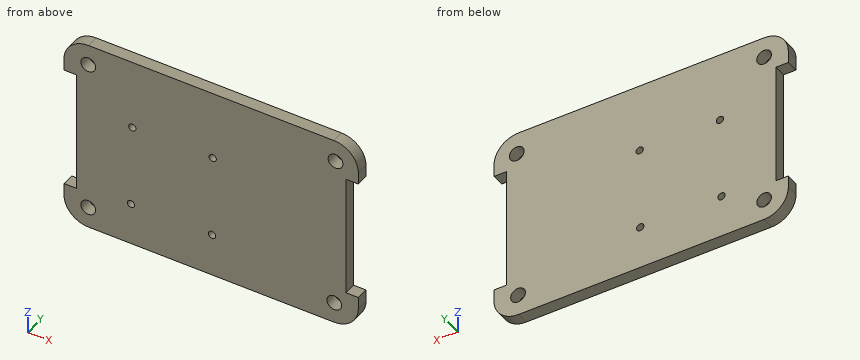
from build123d import *

# Parameters (mm, degrees)
BOSS_EXTRUDE1_DEPTH = 5
SKETCH2_R           = 3
SKETCH2_R_2         = 3.002001364
SKETCH2_R_3         = 2.999925667
SKETCH2_R_4         = 2.998527559
CUT_EXTRUDE2_DEPTH  = 5
SKETCH14_R          = 1.488706827
SKETCH14_R_2        = 1.489546346
SKETCH14_R_3        = 1.489389331
SKETCH14_R_4        = 1.489192683
CUT_EXTRUDE3_DEPTH  = 5


with BuildPart() as part:
    # Sketch1 → Boss-Extrude1 (new body)
    with BuildSketch(Plane(origin=(0, 0, 0), x_dir=(1, 0, 0), z_dir=(0, 1, 0))):
        with BuildLine():
            Line((10, 0), (110, 0))
            ThreePointArc((110, 0), (117.071067812, -2.928932188), (120, -10))
            Line((120, -10), (120, -15))
            Line((120, -15), (115, -15))
            Line((115, -15), (115, -65))
            Line((115, -65), (120, -65))
            Line((120, -65), (120, -70))
            ThreePointArc((120, -70), (117.071067812, -77.071067812), (110, -80))
            Line((110, -80), (10, -80))
            ThreePointArc((10, -80), (2.928932188, -77.071067812), (0, -70))
            Line((0, -70), (0, -65))
            Line((0, -65), (5, -65))
            Line((5, -65), (5, -15))
            Line((5, -15), (0, -15))
            Line((0, -15), (0, -10))
            ThreePointArc((0, -10), (2.928932188, -2.928932188), (10, 0))
        make_face()
    extrude(amount=BOSS_EXTRUDE1_DEPTH)

    # Sketch2 → Cut-Extrude2 (cut)
    with BuildSketch(Plane(origin=(0, 5, 0), x_dir=(1, 0, 0), z_dir=(0, 1, 0))):
        with Locations((9.871405569, -8.58955783)):
            Circle(SKETCH2_R)
        with Locations((9.87978839, -71.481609293)):
            Circle(SKETCH2_R_2)
        with Locations((110.711521692, -71.131223036)):
            Circle(SKETCH2_R_3)
        with Locations((110.199519212, -8.625779617)):
            Circle(SKETCH2_R_4)
    extrude(amount=-CUT_EXTRUDE2_DEPTH, mode=Mode.SUBTRACT)

    # Sketch14 → Cut-Extrude3 (cut)
    with BuildSketch(Plane(origin=(0, 5, 0), x_dir=(1, 0, 0), z_dir=(0, 1, 0))):
        with Locations((27.278668434, -17.438830443)):
            Circle(SKETCH14_R)
        with Locations((60.371161684, -17.660103474)):
            Circle(SKETCH14_R_2)
        with Locations((27.872388447, -51.343688287)):
            Circle(SKETCH14_R_3)
        with Locations((60.628260138, -51.620538185)):
            Circle(SKETCH14_R_4)
    extrude(amount=-CUT_EXTRUDE3_DEPTH, mode=Mode.SUBTRACT)


solid = part.part
Source: CAD feature listing. Evaluate the final solid. Frame: model axes, mm. Round coordinates to 2 decimals unless told otherwise and drop trailing zeros. Loops run counter-clockwise (first coordinate to the right, second up) from the corner with the lowest first, then second, coordinate; pieces in that order, holes last. Notation, with made-up numbers: (16.25, 73) - (22.25, 73) arc R10 cw to (22.25, 91) - close; hole circle Ø9 at (9.25, -21). An arc over 180 degrees is marked (long way). Write item = value, one per line. Start each with the question number.
Item 1: Section query A-A on y = 4.2. Count the separate pieces of the cut face and the enclosed holes in it, plus the area to 3 significant figures.
Item 2: Material intervals for line 1 (X direction, y = 4.05, z = 71); line 2 (X direction, y = 0.9, z = 35); line 3 (Z direction, x = 110, y = 3.7), sorted ascending.
Item 3: Section query B-B on z = 63.5. Output: boundary loops of the cut face in (x, y).
Item 4: First-contact query: pin 1 Ø2 at (y, z) = (3, 71) entering from +X; pin 2 Ø2.5 at (y, z) = (2.5, 48) entering from +X; pin 3 Ø1.5 at (y, z) = (1.5, 32.5) entering from -X; pin 4 Ø1.5 at (x, y) = (2.5, 1.5) entering from -Z. Flat tips, straight axial feed; report the tip coordinate or a pass-through.
Results list:
q1.separate_pieces = 1
q1.enclosed_holes = 8
q1.area = 8,870 mm²
q2.line_1 = 0.05 to 6.92, 12.84 to 107.71, 113.71 to 119.95
q2.line_2 = 5 to 115
q2.line_3 = 0 to 5.63, 11.62 to 68.22, 74.05 to 80
q3.outline = (5, 0) - (115, 0) - (115, 5) - (5, 5) - close
q4.pin_1 = 120
q4.pin_2 = 115
q4.pin_3 = 5
q4.pin_4 = 2.62
